from build123d import *

# Parameters (mm, degrees)
F0_W     = 49.5728366077
F0_H     = 49.0062981844
F1_DEPTH = 79.9
F2_W     = 49.5728366077
F2_H     = 8.2149282098
F3_DEPTH = 45
F4_R     = 10
F5_R     = 5
F7_W     = 52.4731706828
F7_H     = 27.6486203074
F8_DEPTH = 44


with BuildPart() as f1:
    # F0 (on Front) → F1 (new body)
    with BuildSketch(Plane.XZ):
        Rectangle(F0_W, F0_H)
    extrude(amount=-F1_DEPTH)

    # F2 (on face) → F3 (join)
    with BuildSketch(Plane(origin=(0, 79.9, 0), x_dir=(-1, 0, 0), z_dir=(0, 1, 0))):
        with Locations((0, -20.3956849873)):
            Rectangle(F2_W, F2_H)
    extrude(amount=F3_DEPTH)

    # F4
    f4_edges = [f1.edges().sort_by_distance(p)[0] for p in [
        (0, 0, 24.503149),
    ]]
    fillet(f4_edges, radius=F4_R)

    # F5
    f5_edges = [f1.edges().sort_by_distance(p)[0] for p in [
        (24.786418, 2.928932, 21.574217),
        (-24.786418, 2.928932, 21.574217),
    ]]
    fillet(f5_edges, radius=F5_R)

    # F7 (on face) → F8 (cut)
    with BuildSketch(Plane.YZ.offset(24.7864183038)):
        with Locations((43.3237338439, -0.006724149)):
            Rectangle(F7_W, F7_H)
    extrude(amount=-F8_DEPTH, mode=Mode.SUBTRACT)


solid = f1.part
For this review, take the finished solid that the model builds, in its own axes (mm). A direction names the side the tool comes from. Round coordinates to 2 decimals unless told otherwise and drop trailing zeros. Order: outer loops, then holes, each group sorted by start corner. A loop starts at its lowest first (then second) coordinate and runs counter-clockwise, first axis right, second up. Notation, with made-up numbers: (17.25, 23) -> (44.25, 23) arc R14 ccw to (44.25, 31) -> close; hole circle Ø8 at (-11, -36.75). An arc over 180 degrees is marked (long way). Write item = value, one per line. Start each with the question number.
1) Take a section at D-D on y = 81.5. State the section outline as (x, z) points.
2) Take a section at A-A on x = -10. State the section outline as (y, z) points.
3) To check wall thickness, follow line 1 (Z direction, x = -1.5, y = 67.5); line 2 (Y direction, x = 8.5, z = -5.5); line 3 (Z direction, x = 1.5, y = 84.5). State the ranges of each line that lie inside material, in increasing order. Write a range as from..to.
4) Tool access review of faces 1 (the face through (0, 79.9, 4)), 2 (the face through (-24.786, 51, -3)), 3 (the face through (3, 69.56, 0)): name each direction out of +Z, -Z, +X, -X, +Y, -Y from which nothing blocks a thin tool from reaching the whole face with its end or side.
5) The part is to be moulded in two halves that separate along Y. For faces 4 (the face through (3, 17.087, 0)), 5 (the face through (0, 0, -5)), 6 (the face through (-23.28, 45.44, 23.08)), say which applies: +Y half, -Y half, draft (parallel to the pull), parting line (faces both ways), or undercut.
6) Take a section at C-C on y = 52. State the section outline as (x, z) points.
7) Take a section at B-B on z = 12.5. State the section outline as (x, y) points.
8) Insertion check: pin 1 (10 mm diameter, centred on y = 55.5, z = 6.5, fed in from +X); pin 2 (20.5 mm diameter, centred on x = 9.5, z = 13, fed in from +Y); pin 3 (4 mm diameter, centred on x = 12, z = 19, fed in from -Y). Each pin has a flat end and moves straight along its axis. Give the tip position at first contact, or say it passes through.
Verdict:
q1.outline = (-24.79, -24.5) -> (24.79, -24.5) -> (24.79, -16.29) -> (-24.79, -16.29) -> close
q2.outline = (0, -24.5) -> (124.9, -24.5) -> (124.9, -16.29) -> (79.9, -16.29) -> (79.9, 24.5) -> (10, 24.5) arc R10 ccw to (0, 14.5) -> close; hole (17.09, -13.83) -> (69.56, -13.83) -> (69.56, 13.82) -> (17.09, 13.82) -> close
q3.line_1 = -24.5..-13.83, 13.82..24.5
q3.line_2 = 0..17.09, 69.56..79.9
q3.line_3 = -24.5..-16.29
q4.face_1 = +Z, +X, -X, +Y
q4.face_2 = +Z, -Z, -X, +Y, -Y
q4.face_3 = +X
q5.face_4 = undercut
q5.face_5 = -Y half
q5.face_6 = draft
q6.outline = (-24.79, -24.5) -> (24.79, -24.5) -> (24.79, -13.83) -> (-19.21, -13.83) -> (-19.21, 13.82) -> (24.79, 13.82) -> (24.79, 19.5) arc R5 ccw to (19.79, 24.5) -> (-19.79, 24.5) arc R5 ccw to (-24.79, 19.5) -> close
q7.outline = (-24.79, 5) arc R5 ccw to (-19.79, 0) -> (19.79, 0) arc R5 ccw to (24.79, 5) -> (24.79, 17.09) -> (-19.21, 17.09) -> (-19.21, 69.56) -> (24.79, 69.56) -> (24.79, 79.9) -> (-24.79, 79.9) -> close
q8.pin_1 = -19.21
q8.pin_2 = 79.9
q8.pin_3 = 0.32
